Can you work these out from the model? Positions are in its coordinate system, mm. Face numbers are marked on the shaded views. A direction names the side the tool comes from. Round coordinates to 2 decimals unless told otherwise and drop trailing zeros. Order: outer loops, then holes, each group sorted by start corner. A loop starts at its lowest first (then second) coordinate and runs counter-clockwise, first axis right, second up. Notation, with made-up numbers: M -24.5,-36 L -19.5,-36 A28 ccw -19.5,-17 Z; hole C -29,71.25 d9. An arc over 180 degrees is marked long. Answer as a JSON object with one key per item and string values. Group by question number.
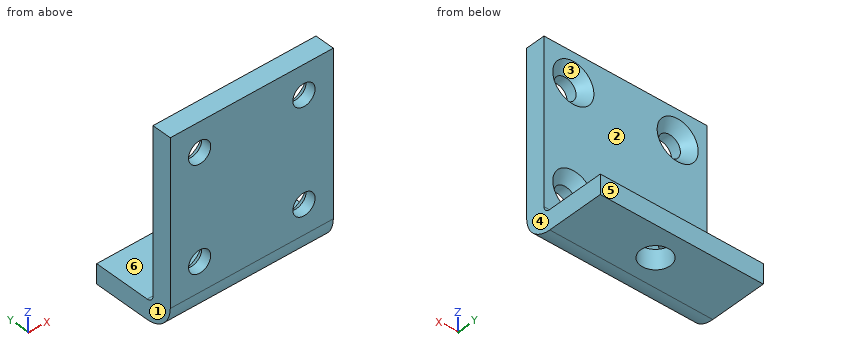
from build123d import *

# Parameters (mm, degrees)
T_LE_DE_BASE_PLI_E1_DEPTH                   = 25
FRAISAGE_POUR_VIS_T_TE_FRAIS_E_M31_AT_COUNT = 2
FRAISAGE_POUR_VIS_T_TE_FRAIS_E_M31_AT_PITCH = 16
FRAISAGE_POUR_VIS_T_TE_FRAIS_E_M31_2_COUNT  = 2
FRAISAGE_POUR_VIS_T_TE_FRAIS_E_M31_2_PITCH  = 22.627416998
FRAISAGE_POUR_VIS_T_TE_FRAIS_E_M31_3_COUNT  = 2
FRAISAGE_POUR_VIS_T_TE_FRAIS_E_M31_3_PITCH  = 16
D_GAGEMENT_M41_D                            = 4.5


# Sheet-metal steps are written as plain solids
with BuildPart() as part:
    # Esquisse1 → Tôle de base pliée1 (new body)
    with BuildSketch(Plane(origin=(0, 0, 0), x_dir=(0, 0, -1), z_dir=(1, 0, 0))):
        with BuildLine():
            Line((0, 12.75), (0, 4))
            ThreePointArc((0, 4), (-1.171572875, 1.171572875), (-4, 0))
            Line((-4, 0), (-29, 0))
            Line((-29, 0), (-29, 3))
            Line((-29, 3), (-4, 3))
            ThreePointArc((-4, 3), (-3.292893219, 3.292893219), (-3, 4))
            Line((-3, 4), (-3, 12.75))
            Line((-3, 12.75), (0, 12.75))
        make_face()
    extrude(amount=T_LE_DE_BASE_PLI_E1_DEPTH)

    # Esquisse7 → Fraisage pour vis à tête fraisée M31 (revolve, cut)
    with BuildSketch(Plane(origin=(4.5, 3, 24.5), x_dir=(0, 0, 1), z_dir=(1, 0, 0))):
        Polygon((0, 0), (0, 3), (1.7, 3), (1.7, 1.45), (3.15, 0), align=None)
    fraisage_pour_vis_t_te_frais_e_m31 = revolve(axis=Axis((4.5, 9.35, 24.5), (0, -1, 0)), mode=Mode.SUBTRACT)

    # Fraisage pour vis à tête fraisée M31 at: Fraisage pour vis à tête fraisée M31 ×2
    with Locations(*[(0, 0, -i * FRAISAGE_POUR_VIS_T_TE_FRAIS_E_M31_AT_PITCH) for i in range(1, FRAISAGE_POUR_VIS_T_TE_FRAIS_E_M31_AT_COUNT)]):
        add(fraisage_pour_vis_t_te_frais_e_m31, mode=Mode.SUBTRACT)

    # Fraisage pour vis _ t_te frais_e M31 2: Fraisage pour vis à tête fraisée M31 ×2
    with Locations(*[Vector(0.7071067811865476, 0, -0.7071067811865476) * (i * FRAISAGE_POUR_VIS_T_TE_FRAIS_E_M31_2_PITCH) for i in range(1, FRAISAGE_POUR_VIS_T_TE_FRAIS_E_M31_2_COUNT)]):
        add(fraisage_pour_vis_t_te_frais_e_m31, mode=Mode.SUBTRACT)

    # Fraisage pour vis _ t_te frais_e M31 3: Fraisage pour vis à tête fraisée M31 ×2
    with Locations(*[(i * FRAISAGE_POUR_VIS_T_TE_FRAIS_E_M31_3_PITCH, 0, 0) for i in range(1, FRAISAGE_POUR_VIS_T_TE_FRAIS_E_M31_3_COUNT)]):
        add(fraisage_pour_vis_t_te_frais_e_m31, mode=Mode.SUBTRACT)

    # Dégagement M41 (through all)
    with Locations(Plane.XY.offset(3)):
        with Locations((12.5, 8.2)):
            Hole(D_GAGEMENT_M41_D / 2)


solid = part.part
Item 1: I'm going to push flat-ended pins straight in: pin 1 Ø5.5 at (x, z) = (20.5, 8.5) entering from +Y; pin 2 Ø4.5 at (x, y) = (18.5, 7.5) entering from +Z; pin 3 Ø10 at (x, z) = (3, 16) entering from +Y. Where does each tip first touch, or does it pass through?
Item 2: If we mould it in two halves opening along X, with no side actions, what happens to the marked faces 1, 2, 3 and 4? For each: +X half, -X half, draft (parallel to the pull), parting line (faces both ways), or undercut.
Item 3: Suppose I cut it at A-A, the plane x = 12.5. Write out the boundary of the cut face in (y, z).
Item 4: I need wall thicknesses on line 1 (X direction, y = 0.5, z = 8.5); line 2 (Z direction, x = 4.5, y = 1.15); line 3 (Z direction, x = 4.5, y = 0.65). Which ranges of each line are inside material? Lowest first, please.
Item 5: On a 3-axis mill with a long thin cutter (end or side, diameter ignored), from which of +Z, -Z, +X, -X, +Y, -Y can I reach the whole of each face in a straight line? I mean the marked faces 5 and 6. Say none if no direction works.
Item 6: Suppose I cut it at C-C, the plane y = 9.25. Write out the boundary of the cut face in (x, z).
Item 7: Suppose I cut it at D-D, the plane x = 4.5. Write out the boundary of the cut face in (y, z).
Item 8: Suppose I cut it at B-B, the plane z = 24.5. Write out the boundary of the cut face in (x, y), and give its area (3 significant figures).
Computed:
{
 "1": {"pin 1": "stops at y = 2.6", "pin 2": "stops at z = 3", "pin 3": "stops at y = 3"},
 "2": {"face 1": "-X half", "face 2": "draft", "face 3": "undercut", "face 4": "+X half"},
 "3": {"outline": "M 0,4 A4 ccw 4,0 L 5.95,0 L 5.95,3 L 4,3 A1 cw 3,4 L 3,29 L 0,29 Z; M 10.45,0 L 12.75,0 L 12.75,3 L 10.45,3 Z"},
 "4": {"line 1": "x = 0 to 2.8, 6.2 to 18.8, 22.2 to 25", "line 2": "z = 1.19 to 6.8, 10.2 to 22.8, 26.2 to 29", "line 3": "z = 1.81 to 6.8, 10.2 to 22.8, 26.2 to 29"},
 "5": {"face 5": "+Z, -Z, +X, -X, +Y", "face 6": "+Z, +X, -X, +Y"},
 "6": {"outline": "M 0,0 L 10.51,0 L 10.51,3 L 0,3 Z; M 14.49,0 L 25,0 L 25,3 L 14.49,3 Z"},
 "7": {"outline": "M 0,4 A4 ccw 4,0 L 12.75,0 L 12.75,3 L 4,3 A1 cw 3,4 L 3,5.35 L 1.55,6.8 L 0,6.8 Z; M 0,10.2 L 1.55,10.2 L 3,11.65 L 3,21.35 L 1.55,22.8 L 0,22.8 Z; M 0,26.2 L 1.55,26.2 L 3,27.65 L 3,29 L 0,29 Z"},
 "8": {"outline": "M 0,0 L 2.8,0 L 2.8,1.55 L 1.35,3 L 0,3 Z; M 6.2,0 L 18.8,0 L 18.8,1.55 L 17.35,3 L 7.65,3 L 6.2,1.55 Z; M 22.2,0 L 25,0 L 25,3 L 23.65,3 L 22.2,1.55 Z", "area": "50.4 mm^2"}
}
